from build123d import *

# Parameters (mm, degrees)
SKETCH2_W               = 57.573593128
SKETCH2_H               = 35
BOSS_EXTRUDE1_DEPTH     = 140
CUT_EXTRUDE1_DEPTH      = 65
CUT_EXTRUDE1_DEPTH_BACK = 65
SKETCH4_W               = 55
SKETCH4_H               = 35
CUT_EXTRUDE2_DEPTH      = 5
CUT_EXTRUDE3_DEPTH      = 161.923336852
BOSS_EXTRUDE2_START     = -135
BOSS_EXTRUDE2_DEPTH     = 10
BOSS_EXTRUDE2_START_2   = -15
BOSS_EXTRUDE2_2_DEPTH   = 10
SKETCH8_3_W             = 10
SKETCH8_3_H             = 10
BOSS_EXTRUDE3_DEPTH     = 30
SKETCH7_R               = 3.125
SKETCH7_R_2             = 1.5
CUT_EXTRUDE5_DEPTH      = 33
SKETCH7_4_R             = 1.5
CUT_EXTRUDE6_DEPTH      = 35


# Read off the part's stored shape, not the designer's step: Boss-Extrude2
with BuildPart() as part:
    # Sketch2 → Boss-Extrude1 (new body)
    with BuildSketch(Plane(origin=(0, 0, 0), x_dir=(0, 0, -1), z_dir=(1, 0, 0))):
        Polygon((-28.786796564, 17.5), (-71.213203436, -17.5), (-28.786796564, -17.5), align=None)
        Rectangle(SKETCH2_W, SKETCH2_H)
        Polygon((-26.990568975, 12.5), (-28.786796564, 11.018187839), (-28.786796564, -17.5), (23.786796564, -17.5), (23.786796564, 12.5), align=None)
        Polygon((-28.786796564, -17.5), (-28.786796564, 11.018187839), (-63.356060578, -17.5), align=None)
    extrude(amount=-BOSS_EXTRUDE1_DEPTH)

    # Sketch3 → Cut-Extrude1 (cut, two sides: drawn at the far end of the back side and taken through both)
    with BuildSketch(Plane.ZY.offset(70).offset(-CUT_EXTRUDE1_DEPTH_BACK)):
        Polygon((-23.786796564, -17.5), (-23.786796564, 12.5), (26.990568975, 12.5), (63.356060578, -17.5), align=None)
    extrude(amount=CUT_EXTRUDE1_DEPTH + CUT_EXTRUDE1_DEPTH_BACK, mode=Mode.SUBTRACT)

    # Sketch4 → Cut-Extrude2 (cut)
    with BuildSketch(Plane(origin=(0, 24.544202322, 20.247933884), x_dir=(1, 0, 0), z_dir=(0, 0.77138921583987, 0.6363636363636365))):
        with Locations((-87.5, -38.569460792)):
            Rectangle(SKETCH4_W, SKETCH4_H)
    extrude(amount=-CUT_EXTRUDE2_DEPTH, mode=Mode.SUBTRACT)

    # Sketch6 → Cut-Extrude3 (cut, through all)
    with BuildSketch(Plane.XZ.offset(17.5)):
        with BuildLine():
            Line((-140, 61.213203436), (-140, 71.213203436))
            Line((-140, 71.213203436), (-130, 71.213203436))
            ThreePointArc((-130, 71.213203436), (-137.071067812, 68.284271247), (-140, 61.213203436))
        make_face()
        with BuildLine():
            Line((-140, -18.786796564), (-140, -28.786796564))
            Line((-140, -28.786796564), (-130, -28.786796564))
            ThreePointArc((-130, -28.786796564), (-137.071067812, -25.857864376), (-140, -18.786796564))
        make_face()
    extrude(amount=-CUT_EXTRUDE3_DEPTH, mode=Mode.SUBTRACT)

    # Boss-Extrude2 outline → Boss-Extrude2 (add)
    with BuildSketch(Plane.YZ.offset(BOSS_EXTRUDE2_START)):
        Polygon((-9.250420886, 53.356060578), (-17.5, 63.356060578), (-17.5, 53.356060578), align=None)
    extrude(amount=BOSS_EXTRUDE2_DEPTH)

    # Boss-Extrude2 2 outline → Boss-Extrude2 2 (add)
    with BuildSketch(Plane.YZ.offset(BOSS_EXTRUDE2_START_2)):
        Polygon((-9.250420886, 53.356060578), (-17.5, 63.356060578), (-17.5, 53.356060578), align=None)
    extrude(amount=BOSS_EXTRUDE2_2_DEPTH)

    # Sketch8<3> → Boss-Extrude3 (add)
    with BuildSketch(Plane.XZ.offset(17.5)):
        with Locations((-130, -18.786796564)):
            Rectangle(SKETCH8_3_W, SKETCH8_3_H)
        with Locations((-10, -18.786796564)):
            Rectangle(SKETCH8_3_W, SKETCH8_3_H)
    extrude(amount=-BOSS_EXTRUDE3_DEPTH)

    # Sketch7 → Cut-Extrude5 (cut)
    # profile 1 of 4: a face of its own
    with BuildSketch(Plane(origin=(0, 17.5, 0), x_dir=(1, 0, 0), z_dir=(0, 1, 0))):
        with Locations(Location((-133, 21.786796564, 0), (0, 0, 270))):
            Circle(SKETCH7_R)
        with Locations(Location((-133, 21.786796564, 0), (0, 0, 270))):
            Circle(SKETCH7_R_2, mode=Mode.SUBTRACT)
    # profile 2 of 4: a face of its own
    with BuildSketch(Plane(origin=(0, 17.5, 0), x_dir=(1, 0, 0), z_dir=(0, 1, 0))):
        with Locations(Location((-7, 21.786796564, 0), (0, 0, 270))):
            Circle(SKETCH7_R)
        with Locations(Location((-7, 21.786796564, 0), (0, 0, 270))):
            Circle(SKETCH7_R_2, mode=Mode.SUBTRACT)
    # profile 3 of 4: a face of its own
    with BuildSketch(Plane(origin=(0, 17.5, 0), x_dir=(1, 0, 0), z_dir=(0, 1, 0))):
        with Locations(Location((-7, -64.213203436, 0), (0, 0, 90))):
            Circle(SKETCH7_R)
        with Locations(Location((-7, -64.213203436, 0), (0, 0, 90))):
            Circle(SKETCH7_R_2, mode=Mode.SUBTRACT)
    # profile 4 of 4: a face of its own
    with BuildSketch(Plane(origin=(0, 17.5, 0), x_dir=(1, 0, 0), z_dir=(0, 1, 0))):
        with Locations(Location((-133, -64.213203436, 0), (0, 0, 90))):
            Circle(SKETCH7_R)
        with Locations(Location((-133, -64.213203436, 0), (0, 0, 90))):
            Circle(SKETCH7_R_2, mode=Mode.SUBTRACT)
    extrude(amount=-CUT_EXTRUDE5_DEPTH, mode=Mode.SUBTRACT)

    # Sketch7<4> → Cut-Extrude6 (cut)
    with BuildSketch(Plane(origin=(0, 17.5, 0), x_dir=(1, 0, 0), z_dir=(0, 1, 0))):
        with Locations(Location((-133, -64.213203436, 0), (0, 0, 90))):
            Circle(SKETCH7_4_R)
        with Locations(Location((-133, 21.786796564, 0), (0, 0, 90))):
            Circle(SKETCH7_4_R)
        with Locations(Location((-7, 21.786796564, 0), (0, 0, 90))):
            Circle(SKETCH7_4_R)
        with Locations(Location((-7, -64.213203436, 0), (0, 0, 90))):
            Circle(SKETCH7_4_R)
    extrude(amount=-CUT_EXTRUDE6_DEPTH, mode=Mode.SUBTRACT)


solid = part.part
Work out the finished part from the listing and answer in its coordinate system (mm). A direction names the side the tool comes from. Round coordinates to 2 decimals unless told otherwise and drop trailing zeros. Loops run counter-clockwise (first coordinate to the right, second up) from the corner with the lowest first, then second, coordinate; pieces in that order, holes last. Notation, with made-up numbers: (5, 21) - (18, 21) arc R17 cw to (18, 28) - close; hole circle Ø11 at (-1, 39.5). An arc over 180 degrees is marked (long way). Use one line per item in the form item = value. Start each with the question number.
(1) Determine the mould class of faces 4 (the face through (-15, -15, 56)), 5 (the face through (-64, 0, -28.787)), 6 (the face through (-140, 0, 13)) for opening direction X: +X half, -X half, draft (parallel to the pull), parting line (faces both ways), or undercut.
(2) Find section B-B on z = 50. Determine the outline of the cut face in (x, y), and give its area (3 significant figures).
(3) Flat-ended cylindrical pins translate along their axes: P1, Ø6.5, axis at y = -14, z = 57, coming from the +X side; P2, Ø8, axis at x = -45.5, y = -3, coming from the +Z side; P3, Ø5, axis at x = -133, z = 64.21, coming from the +Y side; P4, Ø1.8, axis at x = -7, z = 64.21, coming from the -Y side. Find the tip coordinate at first contact, or state that the pin passes through.
(4) Find section C-C on y = -5.5. Determine the outline of the cut face in (x, z) (3 decimals).
(5) Which of the six approach directions +Z, -Z, +X, -X, +Y, -Y give full straight-line access (tool end or side, diameter ignored) to faces 1 (the face through (-69, 17.5, 0)), 2 (the face through (-130, -3, -13.787)), 3 (the face through (-136.05, 1.23, -22.46))?
(6) Find section A-A on x = -66. Determine the outline of the cut face in (y, z), and give its area (3 significant figures).
(7) Consider line 1 (X direction, y = 3.5, z = 16); line 2 (X direction, y = 0, z = 46.5); line 3 (Z direction, x = -7, y = -16.75). Determine where each line is inside the solid, lowest interval first.
(8) Find section D-D on x = -7. Determine the outline of the cut face in (y, z).
Answer list:
q1.face_4 = undercut
q1.face_5 = draft
q1.face_6 = -X half
q2.outline = (-140, -17.5) - (-135, -17.5) - (-135, -6.48) - (-115, -6.48) - (-115, 0) - (-140, 0) - close; (-60, -6.48) - (-5, -6.48) - (-5, -17.5) - (0, -17.5) - (0, 0) - (-60, 0) - close
q2.area = 661 mm^2
q3.P1 = 0
q3.P2 = 58.49
q3.P3 = -15.5
q3.P4 = through
q4.outline = (-140, -18.787) arc R10 ccw to (-130, -28.787) - (0, -28.787) - (0, 56.667) - (-60, 56.667) - (-60, 48.81) - (-5, 48.81) - (-5, -13.787) - (-15, -13.787) - (-15, -23.787) - (-125, -23.787) - (-125, -13.787) - (-135, -13.787) - (-135, 48.81) - (-115, 48.81) - (-115, 56.667) - (-140, 56.667) - close; hole circle Ø6.25 at (-133, -21.787); hole circle Ø6.25 at (-7, -21.787)
q5.face_1 = +Z, -Z, +X, -X, +Y
q5.face_2 = -Y
q5.face_3 = +Y
q6.outline = (-17.5, -28.79) - (17.5, -28.79) - (17.5, 28.79) - (11.14, 36.5) - (7.28, 33.32) - (12.5, 26.99) - (12.5, -23.79) - (-17.5, -23.79) - close; (-17.5, 63.36) - (-14.99, 60.32) - (-11.14, 63.5) - (-17.5, 71.21) - close
q6.area = 514 mm^2
q7.line_1 = -140 to -135, -5 to 0
q7.line_2 = -140 to -115, -60 to 0
q7.line_3 = -28.79 to -23.29, -20.29 to -13.79, 53.36 to 62.71, 65.71 to 70.3
q8.outline = (-17.5, -28.79) - (17.5, -28.79) - (17.5, -24.91) - (-15.5, -24.91) - (-15.5, -23.29) - (-17.5, -23.29) - close; (-17.5, -20.29) - (-15.5, -20.29) - (-15.5, -18.66) - (17.5, -18.66) - (17.5, 28.79) - (-9.15, 61.09) - (-15.5, 61.09) - (-15.5, 62.71) - (-17.5, 62.71) - (-17.5, 53.36) - (-9.25, 53.36) - (12.5, 26.99) - (12.5, -13.79) - (-17.5, -13.79) - close; (-17.5, 65.71) - (-15.5, 65.71) - (-15.5, 67.34) - (-14.3, 67.34) - (-17.5, 71.21) - close
